Geometry check sheet. Reference: the model listing, model coordinates, mm. Face numbers are marked on the shaded views. Round coordinates to 2 decimals unless told otherwise and drop trailing zeros. Loops run counter-clockwise (first coordinate to the right, second up) from the corner with the lowest first, then second, coordinate; pieces in that order, holes last. Notation, with made-up numbers: (-14, 58.25) - (40, 58.25) arc R14 ccw to (40, 79.25) - close; hole circle Ø4 at (27, 88.25). An arc over 180 degrees is marked (long way). Write item = value, one per line.
```python
from build123d import *

# Parameters (mm, degrees)
F1_DEPTH = 35
F2_R     = 5
F3_SIZE  = 2
F4_R     = 2.5
F4_R_2   = 1.5
F5_DEPTH = 5


with BuildPart() as f1:
    # F0 (on Right) → F1 (new body)
    with BuildSketch(Plane.YZ):
        with BuildLine():
            ThreePointArc((12, -0.8728863157), (8.4852813742, 7.6123950585), (0, 11.1271136843))
            Line((0, 11.1271136843), (0, 5.1271136843))
            ThreePointArc((0, 5.1271136843), (4.2426406871, 3.3697543714), (6, -0.8728863157))
            ThreePointArc((6, -0.8728863157), (4.2426406871, -5.1155270029), (0, -6.8728863157))
            Line((0, -6.8728863157), (0, -12.8728863157))
            ThreePointArc((0, -12.8728863157), (8.4852813742, -9.35816769), (12, -0.8728863157))
        make_face()
        with BuildLine():
            Line((0, 5.1271136843), (0, 11.1271136843))
            ThreePointArc((0, 11.1271136843), (-5.6745486619, 9.7006418317), (-10, 5.760363265))
            Line((-10, 5.760363265), (-10, -7.5061358965))
            ThreePointArc((-10, -7.5061358965), (-5.6745486619, -11.4464144632), (0, -12.8728863157))
            Line((0, -12.8728863157), (0, -6.8728863157))
            ThreePointArc((0, -6.8728863157), (-6, -0.8728863157), (0, 5.1271136843))
        make_face()
        with BuildLine():
            Line((-10, -12.8728863157), (0, -12.8728863157))
            ThreePointArc((0, -12.8728863157), (-5.6745486619, -11.4464144632), (-10, -7.5061358965))
            Line((-10, -7.5061358965), (-10, -12.8728863157))
        make_face()
        with BuildLine():
            Line((0, 11.1271136843), (0, 22.1271136843))
            ThreePointArc((0, 22.1271136843), (-5.6745486619, 23.5535855368), (-10, 27.4938641035))
            Line((-10, 27.4938641035), (-10, 5.760363265))
            ThreePointArc((-10, 5.760363265), (-5.6745486619, 9.7006418317), (0, 11.1271136843))
        make_face()
        with BuildLine():
            ThreePointArc((-10, 27.4938641035), (-5.6745486619, 23.5535855368), (0, 22.1271136843))
            ThreePointArc((0, 22.1271136843), (8.4852813742, 25.64183231), (12, 34.1271136843))
            ThreePointArc((12, 34.1271136843), (8.4852813742, 42.6123950585), (0, 46.1271136843))
            ThreePointArc((0, 46.1271136843), (-5.6745486619, 44.7006418317), (-10, 40.760363265))
            Line((-10, 40.760363265), (-10, 27.4938641035))
        make_face()
        with BuildLine():
            ThreePointArc((-6, 34.1271136843), (0, 40.1271136843), (6, 34.1271136843))
            ThreePointArc((6, 34.1271136843), (4.2426406871, 29.8844729971), (0, 28.1271136843))
            ThreePointArc((0, 28.1271136843), (-4.2426406871, 29.8844729971), (-6, 34.1271136843))
        make_face(mode=Mode.SUBTRACT)
        with BuildLine():
            Line((-10, 46.1271136843), (-10, 40.760363265))
            ThreePointArc((-10, 40.760363265), (-5.6745486619, 44.7006418317), (0, 46.1271136843))
            Line((0, 46.1271136843), (-10, 46.1271136843))
        make_face()
    extrude(amount=F1_DEPTH)

    # F2
    f2_edges = [f1.edges().sort_by_distance(p)[0] for p in [
        (17.5, 0, 22.127114),
        (17.5, 0, 11.127114),
    ]]
    fillet(f2_edges, radius=F2_R)

    # F3
    f3_edges = [f1.edges().sort_by_distance(p)[0] for p in [
        (17.5, -10, -12.872886),
        (17.5, -10, 46.127114),
    ]]
    chamfer(f3_edges, length=F3_SIZE)

    # F4 (on face) → F5 (join)
    with BuildSketch(Plane.XZ.offset(10)):
        with Locations((10.5, 24.1271136843)):
            Circle(F4_R)
        with Locations((10.5, 24.1271136843)):
            Circle(F4_R_2, mode=Mode.SUBTRACT)
        with BuildLine():
            ThreePointArc((27, 24.1271136843), (24.5, 26.6271136843), (22, 24.1271136843))
            ThreePointArc((22, 24.1271136843), (24.5, 21.6271136843), (27, 24.1271136843))
        make_face()
        with BuildLine():
            ThreePointArc((26, 24.1271136843), (24.5, 22.6271136843), (23, 24.1271136843))
            ThreePointArc((23, 24.1271136843), (24.5, 25.6271136843), (26, 24.1271136843))
        make_face(mode=Mode.SUBTRACT)
    extrude(amount=F5_DEPTH)


solid = f1.part
```
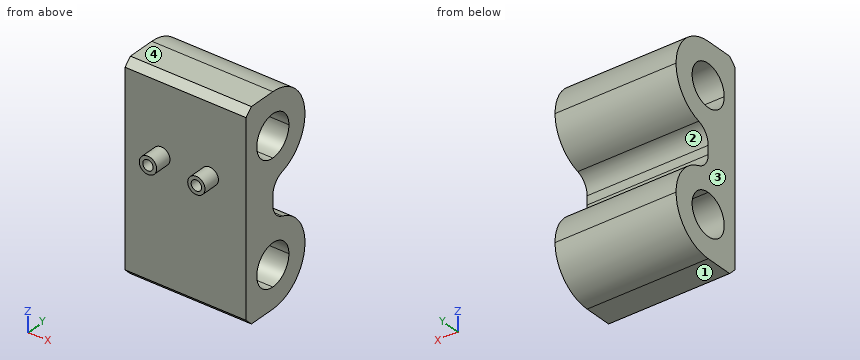
(1) Scan lines: L1, parallel to X at y = -11, z = 24; L2, parallel to Z at x = 10.5, y = -14; L3, parallel to Z at x = 24, y = 4.25. Record each from-to range of solid material in increasing order. Write a range as [from, to].
Answers follow:
L1 = [8, 9.01], [11.99, 13], [22, 23.01], [25.99, 27]
L2 = [21.63, 22.63], [25.63, 26.63]
L3 = [-12.1, -5.11], [3.36, 10.35], [22.9, 29.89], [38.36, 45.35]
(2) Section check B-B (y = 8). Enter the section's corners in (x, z).
Answers follow:
outline = (0, -9.82) - (35, -9.82) - (35, 8.07) - (0, 8.07) - close; (0, 25.18) - (35, 25.18) - (35, 43.07) - (0, 43.07) - close
(3) Mould release check, pull along Z, two halves, no side actions. Record for the marked faces 1, 2, 3 and 4: pulls with the +Z half, pulls with the -Z half, needs draft (parallel to the pull), parting line crosses it, or undercut.
Answers follow:
face_1 = pulls with the -Z half
face_2 = undercut
face_3 = needs draft
face_4 = pulls with the +Z half
(4) Section check C-C (z = 2). Enter the section's corners in (x, y), then the cut area to 3 significant figures.
Answers follow:
outline = (0, -10) - (35, -10) - (35, -5.27) - (0, -5.27) - close; (0, 5.27) - (35, 5.27) - (35, 11.65) - (0, 11.65) - close
area = 389 mm²
(5) Gauge pin test, flat ends, axial feed: pin 1 (4 mm diameter, centred on x = 30.5, z = 29, fed in from -Y); pin 2 (0.8 mm diameter, centred on x = 12, z = 16.5, fed in from +Y); pin 3 (2 mm diameter, centred on x = 27.5, y = 2.5, fed in from +Z). Record the tip position at first contact, or that the pin passes through.
Answers follow:
pin_1 = -10
pin_2 = 0
pin_3 = 46.03
(6) Section check A-A (x = 24.5). Enter the section's corners in (y, z), then the cut area to 3 significant figures.
Answers follow:
outline = (-15, 21.63) - (-10, 21.63) - (-10, -10.87) - (-8, -12.87) - (0, -12.87) arc R12 ccw to (3.53, 10.6) arc R5 cw to (0, 15.38) - (0, 17.88) arc R5 cw to (3.53, 22.66) arc R12 ccw to (0, 46.13) - (-8, 46.13) - (-10, 44.13) - (-10, 26.63) - (-15, 26.63) - (-15, 25.63) - (-10, 25.63) - (-10, 22.63) - (-15, 22.63) - close; hole circle Ø12 at (0, -0.87); hole circle Ø12 at (0, 34.13)
area = 829 mm²
(7) Section check D-D (y = -12.25). Enter the section's corners in (x, z).
Answers follow:
outline = circle Ø5 at (10.5, 24.13); circle Ø5 at (24.5, 24.13); hole circle Ø3 at (10.5, 24.13); hole circle Ø3 at (24.5, 24.13)
